```python
from build123d import *

# Parameters (mm, degrees)
SKETCH1_W                = 140
SKETCH1_H                = 85
BOSS_EXTRUDE1_DEPTH      = 18
SKETCH2_W                = 3
SKETCH2_H                = 49
CUT_EXTRUDE1_DEPTH       = 220
SKETCH3_R                = 8
CUT_EXTRUDE4_DEPTH       = 30
SKETCH5_W                = 56
SKETCH5_H                = 12
BOSS_EXTRUDE2_DEPTH      = 140
BOSS_EXTRUDE3_DEPTH      = 18
BOSS_EXTRUDE3_DEPTH_BACK = 12
SKETCH7_R                = 20
SKETCH8_R                = 9
CUT_EXTRUDE5_DEPTH       = 50
BOSS_EXTRUDE4_DEPTH      = 12
BOSS_EXTRUDE6_DEPTH      = 36
BOSS_EXTRUDE6_DEPTH_BACK = 52
SKETCH11_R               = 27.5
SKETCH12_R               = 15
CUT_EXTRUDE6_DEPTH       = 109
CUT_EXTRUDE11_DEPTH      = 12


with BuildPart() as part:
    # Sketch1 → Boss-Extrude1 (new body)
    with BuildSketch(Plane.XY):
        with Locations((70, -42.5)):
            Rectangle(SKETCH1_W, SKETCH1_H)
    extrude(amount=BOSS_EXTRUDE1_DEPTH)

    # Sketch2 → Cut-Extrude1 (cut)
    with BuildSketch(Plane(origin=(140, 0, 0), x_dir=(0, 0, -1), z_dir=(1, 0, 0))):
        with Locations((-16.5, -42.5)):
            Rectangle(SKETCH2_W, SKETCH2_H)
    extrude(amount=-CUT_EXTRUDE1_DEPTH, mode=Mode.SUBTRACT)

    # Sketch3 → Cut-Extrude4 (cut)
    with BuildSketch(Plane(origin=(0, 0, 0), x_dir=(-1, 0, 0), z_dir=(0, 0, -1))):
        with Locations((-105, -55)):
            Circle(SKETCH3_R)
        with Locations((-30, -55)):
            Circle(SKETCH3_R)
    extrude(amount=-CUT_EXTRUDE4_DEPTH, mode=Mode.SUBTRACT)

    # Sketch5 → Boss-Extrude2 (add)
    with BuildSketch(Plane(origin=(140, 0, 0), x_dir=(0, 0, -1), z_dir=(1, 0, 0))):
        with Locations((10, 6)):
            Rectangle(SKETCH5_W, SKETCH5_H)
    extrude(amount=-BOSS_EXTRUDE2_DEPTH)

    # Sketch7 → Boss-Extrude3 (add, two sides: drawn at the far end of the back side and taken through both)
    with BuildSketch(Plane.XZ.offset(-BOSS_EXTRUDE3_DEPTH_BACK)):
        with Locations(Location((120, -38, 0), (0, 0, 180))):
            Circle(SKETCH7_R)
    extrude(amount=BOSS_EXTRUDE3_DEPTH + BOSS_EXTRUDE3_DEPTH_BACK)

    # Sketch8 → Cut-Extrude5 (cut)
    with BuildSketch(Plane(origin=(0, -18, 0), x_dir=(-1, 0, 0), z_dir=(0, -1, 0))):
        with Locations(Location((-120, 38, 0), (0, 0, 90))):
            Circle(SKETCH8_R)
    extrude(amount=-CUT_EXTRUDE5_DEPTH, mode=Mode.SUBTRACT)

    # Sketch10 → Boss-Extrude4 (add)
    with BuildSketch(Plane.XZ):
        with BuildLine():
            Line((0, -38), (22.5, -100))
            ThreePointArc((22.5, -100), (50, -72.5), (77.5, -100))
            Line((77.5, -100), (120, -58))
            ThreePointArc((120, -58), (105.857864376, -52.142135624), (100, -38))
            Line((100, -38), (0, -38))
        make_face()
    extrude(amount=-BOSS_EXTRUDE4_DEPTH)

    # Sketch11 → Boss-Extrude6 (add, two sides: drawn at the far end of the back side and taken through both)
    with BuildSketch(Plane(origin=(0, 12, 0), x_dir=(1, 0, 0), z_dir=(0, 1, 0)).offset(-BOSS_EXTRUDE6_DEPTH_BACK)):
        with Locations(Location((50, 100, 0), (0, 0, 270))):
            Circle(SKETCH11_R)
    extrude(amount=BOSS_EXTRUDE6_DEPTH + BOSS_EXTRUDE6_DEPTH_BACK)

    # Sketch12 → Cut-Extrude6 (cut)
    with BuildSketch(Plane.XZ.offset(40)):
        with Locations(Location((50, -100, 0), (0, 0, 270))):
            Circle(SKETCH12_R)
    extrude(amount=-CUT_EXTRUDE6_DEPTH, mode=Mode.SUBTRACT)

    # Sketch14 → Cut-Extrude11 (cut)
    with BuildSketch(Plane(origin=(0, 12, 0), x_dir=(1, 0, 0), z_dir=(0, 1, 0))):
        with BuildLine():
            Line((80.968040171, 96.572760302), (116.531959829, 61.427239698))
            ThreePointArc((116.531959829, 61.427239698), (81.177239698, 61.218040171), (80.968040171, 96.572760302))
        make_face()
    extrude(amount=-CUT_EXTRUDE11_DEPTH, mode=Mode.SUBTRACT)


solid = part.part
```
CAD build for the part. Positions are in the model's coordinates, mm. A direction names the side the tool comes from. Round coordinates to 2 decimals unless told otherwise and drop trailing zeros. Write each loop counter-clockwise with the first axis right and the second up, starting at its lowest first coordinate (ties: lowest second). Pieces come first, ordered by that corner, then holes.
Item 1: Mould opens along Y. For faces 1 (the flat face through (38, -40, -88)), 2 (the flat face through (71, -43, 15)), 3 (the cylindrical face through (97.37, -52.6, 7.4)), 4 (the flat face through (0, -25, 3)) say: released by +Y, released by -Y, zero draft, split by the parting line, or undercut.
Filled in:
face 1: released by -Y
face 2: undercut
face 3: undercut
face 4: zero draft
Item 2: Band-saw the part on C-C on y = 4. Write the cut outline in (x, z).
Filled in:
outline: (0, -38) - (22.5, -100) arc R27.5 ccw to (77.5, -100) - (80.97, -96.57) arc R25 cw to (116.53, -61.43) - (120, -58) arc R20 ccw to (140, -38) - (140, 18) - (0, 18) - close; hole circle Ø30 at (50, -100); hole circle Ø18 at (120, -38)
Item 3: Tool access for faces 5 (the flat face through (69, -42, 0)), 6 (the flat face through (116, -18, -29)), 7 (the cylindrical face through (134.74, -6.12, -51.52)): list every direction of +Z, -Z, +X, -X, +Y, -Y with a clear straight run to the whole face (end or side of a thin tool).
Filled in:
face 5: +X, -X, -Y
face 6: -Z, +X, -X, -Y
face 7: -Y
Item 4: Band-saw the part on A-A on y = -27. Write the cut outline in (x, z), then the cut area to 3 significant figures.
Filled in:
outline: (0, 0) - (140, 0) - (140, 15) - (0, 15) - close; circle Ø55 at (50, -100); hole circle Ø30 at (50, -100)
area: 3,770 mm2
Item 5: Band-saw the part on D-D on z = -92. Write the cut outline in (x, y), then the cut area to 3 significant figures.
Filled in:
outline: (19.6, 0) - (23.69, 0) - (23.69, -40) - (37.31, -40) - (37.31, 48) - (23.69, 48) - (23.69, 12) - (19.6, 12) - close; (62.69, -40) - (76.31, -40) - (76.31, 0) - (77.4, 0) - (77.4, 12) - (76.31, 12) - (76.31, 48) - (62.69, 48) - close
area: 2,460 mm2
Item 6: Drill centre lines: L1, parallel to X at y = -26.5, z = -101; L2, parallel to X at y = -8.5, z = -38; L3, parallel to Y at x = 105, z = 11. Where is each one in solid material? Low to high.
Filled in:
L1: x = 22.52 to 35.03, 64.97 to 77.48
L2: x = 100 to 111, 129 to 140
L3: y = -85 to -63, -47 to 12
Item 7: Drop flat-ended pins along their axis: pin 1 Ø14.5 at (x, y) = (101, -54) entering from +Z; pin 2 Ø14.5 at (x, y) = (30, -55) entering from -Z; pin 3 Ø3 at (y, z) = (-8.5, -96.5) entering from -X; pin 4 Ø2 at (x, z) = (48.5, -20.5) entering from +Y. Give the stop position or say it passes through.
Filled in:
pin 1: stops at z = 15
pin 2: passes through
pin 3: stops at x = 22.57
pin 4: stops at y = 12
Item 8: Band-saw the part on B-B on x = 42. Write the cut outline in (y, z).
Filled in:
outline: (-85, 0) - (0, 0) - (0, -73.69) - (-40, -73.69) - (-40, -87.31) - (48, -87.31) - (48, -73.69) - (12, -73.69) - (12, 18) - (-18, 18) - (-18, 15) - (-67, 15) - (-67, 18) - (-85, 18) - close; (-40, -126.31) - (48, -126.31) - (48, -112.69) - (-40, -112.69) - close
